from build123d import *

# Parameters (mm, degrees)
F0_R     = 9
F0_R_2   = 7
F1_DEPTH = 3
F2_DEPTH = 6
F3_R     = 7
F4_DEPTH = 25
F5_R     = 3.75
F6_DEPTH = 4
F7_R     = 7
F8_DEPTH = 9


with BuildPart() as f1:
    # F0 (on Front) → F1 (new body)
    with BuildSketch(Plane.XZ):
        Circle(F0_R)
        Circle(F0_R_2, mode=Mode.SUBTRACT)
        Circle(F0_R_2)
    extrude(amount=F1_DEPTH)

    # F0 (on Front) → F2 (join)
    with BuildSketch(Plane.XZ):
        Circle(F0_R_2)
    extrude(amount=-F2_DEPTH)

    # F3 (on face) → F4 (join)
    with BuildSketch(Plane.XZ.offset(3)):
        Circle(F3_R)
    extrude(amount=F4_DEPTH)

    # F5 (on face) → F6 (join)
    with BuildSketch(Plane.XZ.offset(28)):
        Circle(F5_R)
    extrude(amount=F6_DEPTH)

    # F7 (on face) → F8 (join)
    with BuildSketch(Plane.XZ.offset(32)):
        Circle(F7_R)
    extrude(amount=F8_DEPTH)


solid = f1.part
Build history of the part. All positions in model axes, mm. A direction names the side the tool comes from. Round coordinates to 2 decimals unless told otherwise and drop trailing zeros. Write each loop counter-clockwise with the first axis right and the second up, starting at its lowest first coordinate (ties: lowest second). Pieces come first, ordered by that corner, then holes. Notation, with made-up numbers: M -30.5,-23 L 26.5,-23 A27 ccw 26.5,-6 Z; hole C -36,44.5 d6. An arc over 180 degrees is marked long. Answer as a JSON object with one key per item and string values. Group by question number.
(1) Flat gauge pins, fed straight in: pin 1 (5 mm diameter, centred on y = -31.5, z = 3, fed in from -X); pin 2 (1 mm diameter, centred on y = -23.5, z = 1, fed in from +X); pin 3 (1.5 mm diameter, centred on x = -4.5, y = -0.5, fed in from -Z). Where does each tip first touch, or does it go through?
(2) Drill centre lines: L1, parallel to Y at x = 2.5, z = -5.25; L2, parallel to Y at x = 5.75, z = -6.5; L3, parallel to Z at x = -2, y = 1. Where is each one in solid material? Low to high.
(3) Cut at A-A (x = 0). Give the cut face in (y, z).
(4) Cut at C-C (z = 2.25). Give the cut face in (x, y).
(5) Cut at D-D (y = -31.5). Give the cut face in (x, z).
(6) Cut at B-B (x = 6). Give the cut face in (y, z), and give its area (3 significant figures).
(7) Mould opens along Y. For faces 5 (the flat face through (3, -28, -3)), 6 (the cylindrical face through (6.466, -15.325, -2.681)), 7 (the flat face through (0, -41, 0)), 8 (the flat face through (0, 6, 0)) say: pulls with the +Y half, pulls with the -Y half, needs draft (parallel to the pull), parting line crosses it, or undercut.
(8) Which spindle directions (+Z, -Z, +X, -X, +Y, -Y) get a long thin tool onto all of the face, cutting with end or side? Do faces 1 (the flat face through (0, 0, -7.3)), 2 (the cylindrical face through (-1.172, -1.479, 8.923)), 3 (the cylindrical face through (6.466, -36.437, -2.681)), 4 (the flat face through (3, -32, -3)). Say none if no direction does.
Responses:
{
 "1": {"pin 1": "stops at x = -6.98", "pin 2": "stops at x = 6.98", "pin 3": "stops at z = -8.18"},
 "2": {"L1": "y = -41 to -32, -28 to 6", "L2": "y = -3 to 0", "L3": "z = -6.71 to 6.71"},
 "3": {"outline": "M -41,-7 L -32,-7 L -32,-3.75 L -28,-3.75 L -28,-7 L -3,-7 L -3,-9 L 0,-9 L 0,-7 L 6,-7 L 6,7 L 0,7 L 0,9 L -3,9 L -3,7 L -28,7 L -28,3.75 L -32,3.75 L -32,7 L -41,7 Z"},
 "4": {"outline": "M -8.71,-3 L -6.63,-3 L -6.63,-28 L -3,-28 L -3,-32 L -6.63,-32 L -6.63,-41 L 6.63,-41 L 6.63,-32 L 3,-32 L 3,-28 L 6.63,-28 L 6.63,-3 L 8.71,-3 L 8.71,0 L 6.63,0 L 6.63,6 L -6.63,6 L -6.63,0 L -8.71,0 Z"},
 "5": {"outline": "C 0,0 d7.5"},
 "6": {"outline": "M -41,-3.61 L -32,-3.61 L -32,3.61 L -41,3.61 Z; M -28,-3.61 L -3,-3.61 L -3,-6.71 L 0,-6.71 L 0,-3.61 L 6,-3.61 L 6,3.61 L 0,3.61 L 0,6.71 L -3,6.71 L -3,3.61 L -28,3.61 Z", "area": "329 mm2"},
 "7": {"face 5": "undercut", "face 6": "needs draft", "face 7": "pulls with the -Y half", "face 8": "pulls with the +Y half"},
 "8": {"face 1": "+Y", "face 2": "+Y, -Y", "face 3": "-Y", "face 4": "none"}
}
